Part model, mm, in its own coordinate system. A direction names the side the tool comes from. Round coordinates to 2 decimals unless told otherwise and drop trailing zeros. Write each loop counter-clockwise with the first axis right and the second up, starting at its lowest first coordinate (ties: lowest second). Pieces come first, ordered by that corner, then holes.
from build123d import *

# Parameters (mm, degrees)
SKETCH2_W           = 61
SKETCH2_H           = 20.5
SKETCH2_R           = 1.55
BOSS_EXTRUDE1_DEPTH = 3.175
SKETCH3_W           = 9.85
SKETCH3_H           = 20.5
SKETCH3_R           = 1.55
BOSS_EXTRUDE2_DEPTH = 7.75


with BuildPart() as part:
    # Sketch2 → Boss-Extrude1 (new body)
    with BuildSketch(Plane(origin=(0, 0, 0), x_dir=(1, 0, 0), z_dir=(0, 1, 0))):
        Rectangle(SKETCH2_W, SKETCH2_H)
        with Locations((-24.5, -5)):
            Circle(SKETCH2_R, mode=Mode.SUBTRACT)
        with BuildLine():
            ThreePointArc((-2.233801513, -3), (-17.65, 0), (-2.233801513, 3))
            Line((-2.233801513, 3), (13.766198487, 3))
            Line((13.766198487, 3), (13.766198487, -3))
            Line((13.766198487, -3), (-2.233801513, -3))
        make_face(mode=Mode.SUBTRACT)
        with Locations((24.5, -5)):
            Circle(SKETCH2_R, mode=Mode.SUBTRACT)
        with Locations((-24.5, 5)):
            Circle(SKETCH2_R, mode=Mode.SUBTRACT)
        with Locations((24.5, 5)):
            Circle(SKETCH2_R, mode=Mode.SUBTRACT)
    extrude(amount=BOSS_EXTRUDE1_DEPTH)

    # Sketch3 → Boss-Extrude2 (add)
    with BuildSketch(Plane.XZ):
        with Locations((-25.575, 0)):
            Rectangle(SKETCH3_W, SKETCH3_H)
        with Locations((-24.5, -5)):
            Circle(SKETCH3_R, mode=Mode.SUBTRACT)
        with Locations((-24.5, 5)):
            Circle(SKETCH3_R, mode=Mode.SUBTRACT)
        with Locations((25.575, 0)):
            Rectangle(SKETCH3_W, SKETCH3_H)
        with Locations((24.5, -5)):
            Circle(SKETCH3_R, mode=Mode.SUBTRACT)
        with Locations((24.5, 5)):
            Circle(SKETCH3_R, mode=Mode.SUBTRACT)
    extrude(amount=BOSS_EXTRUDE2_DEPTH)


solid = part.part
Q1. Saw through at C-C, the plane z = 0. Write the cut outline in (x, y) (3 decimals), and give its area (3 significant figures).
Q2. Drop a flat-ended pin along its axis: P1, Ø8, axis at x = 9, z = 3.5, coming from the -Y side. Give the stop position or say it passes through.
Q3. Two-plate mould, pull along X, no slides. Class faces 1 (the flat face through (0, 3.175, -5)), 2 (the cylindrical face through (-17.644, 1.565, 0.309)), 3 (the flat face through (-30.5, -2, 0)): released by +X, released by -X, zero draft, split by the parting line, or undercut.
Q4. Wall check: line 1 (X direction, y = -2.25, z = -5); line 2 (Z direction, x = 24.5, y = -2.75); line 3 (Z direction, x = 13, y = 0.75). Give the ranges that are in metal, low to high.
Q5. Saw through at B-B, the plane y = -5. Write the cut outline in (x, z).
Q6. Tool access for faces 4 (the flat face through (-20.65, -4, 0)), 5 (the flat face through (13.766, 2, 0)), 6 (the flat face through (-0.4, 0.2, 10.25)): list every direction of +Z, -Z, +X, -X, +Y, -Y with a clear straight run to the whole face (end or side of a thin tool).
Q7. Saw through at D-D, the plane x = 24.5. Write the cut outline in (y, z) (3 decimals).
Q8. Saw through at A-A, the plane x = -9.65. Write the cut outline in (y, z) (3 decimals).
Computed:
1. outline: (-30.5, -7.75) - (-20.65, -7.75) - (-20.65, 0) - (-17.65, 0) - (-17.65, 3.175) - (-30.5, 3.175) - close; (13.766, 0) - (20.65, 0) - (20.65, -7.75) - (30.5, -7.75) - (30.5, 3.175) - (13.766, 3.175) - close
1. area: 247 mm2
2. P1: stops at y = 0
3. face 1: zero draft
3. face 2: undercut
3. face 3: released by -X
4. line 1: x = -30.5 to -26.05, -22.95 to -20.65, 20.65 to 22.95, 26.05 to 30.5
4. line 2: z = -10.25 to -6.55, -3.45 to 3.45, 6.55 to 10.25
4. line 3: z = -10.25 to -3, 3 to 10.25
5. outline: (-30.5, -10.25) - (-20.65, -10.25) - (-20.65, 10.25) - (-30.5, 10.25) - close; (20.65, -10.25) - (30.5, -10.25) - (30.5, 10.25) - (20.65, 10.25) - close; hole circle Ø3.1 at (-24.5, -5); hole circle Ø3.1 at (-24.5, 5); hole circle Ø3.1 at (24.5, -5); hole circle Ø3.1 at (24.5, 5)
6. face 4: +Z, -Z, -Y
6. face 5: +Y, -Y
6. face 6: +Z, +X, -X, +Y, -Y
7. outline: (-7.75, -10.25) - (3.175, -10.25) - (3.175, -6.55) - (-7.75, -6.55) - close; (-7.75, -3.45) - (3.175, -3.45) - (3.175, 3.45) - (-7.75, 3.45) - close; (-7.75, 6.55) - (3.175, 6.55) - (3.175, 10.25) - (-7.75, 10.25) - close
8. outline: (0, -10.25) - (3.175, -10.25) - (3.175, -8) - (0, -8) - close; (0, 8) - (3.175, 8) - (3.175, 10.25) - (0, 10.25) - close
